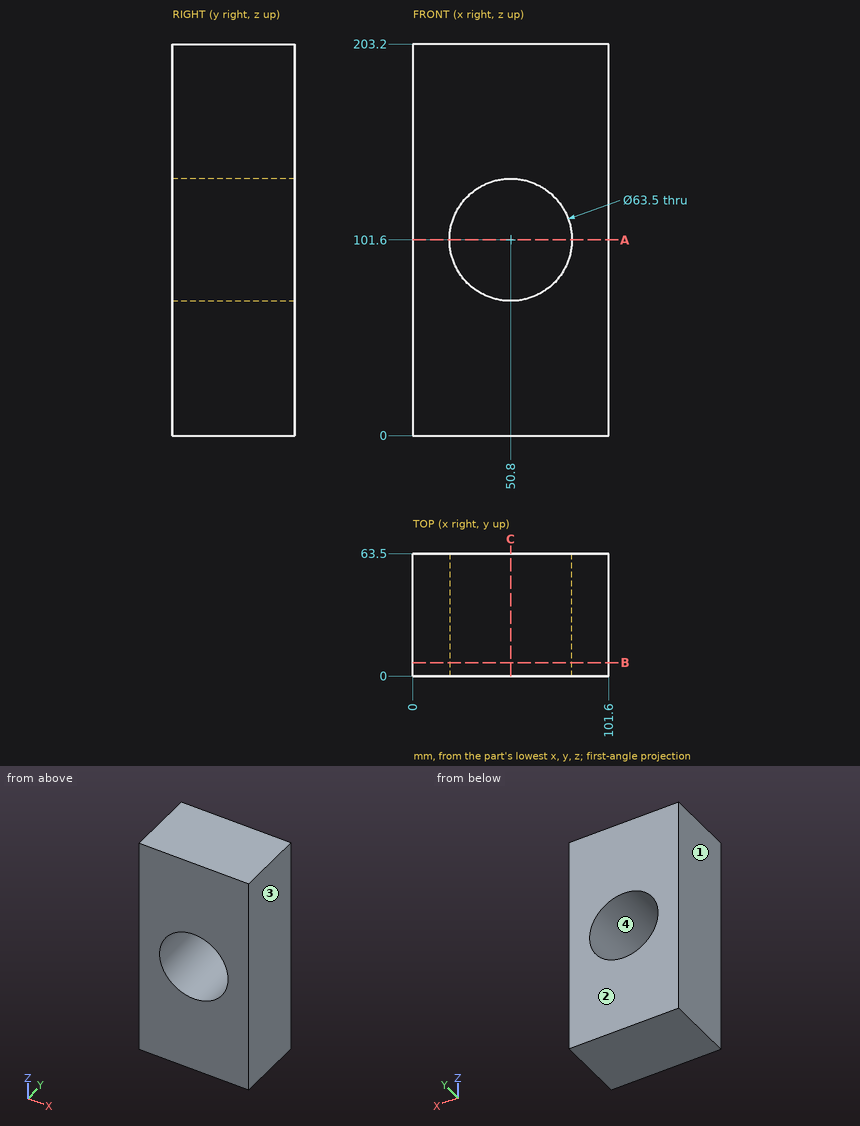
Design review of the part shown in the three views and the two pictorial views. Dimensions are in mm from the part's minimum x, y and z. Give positions to 0.01 mm unless a question says otherwise; leave off trailing zeros. Loops run counter-clockwise (first coordinate to the right, second up) from the corner with the lowest first, then second, coordinate; pieces in that order, holes last. Notation, with made-up numbers: M 31.25,48 L 73.25,48 A18 ccw 73.25,66 Z; hole C 89.25,68 d11. An arc over 180 degrees is marked long. Put each result on its own line as item: value. Start each with the question number.
(1) Wall thickness on L1, parallel to Z at x = 50.8, y = 39; L2, parallel to X at y = 48.5, z = 101.6; L3, parallel to Z at x = 32, y = 10: over which ranges is each line inside the solid? List them lowest first.
(2) Add section B-B, the plane y = 7. Write out the cut boundary in (x, z), then the cut area to 3 significant figures.
(3) For pin 1 (6 mm diameter, centred on x = 27.5, z = 164, fed in from -Y), flat-tipped, find the tip position at first contact; note if it passes through.
(4) Add section C-C, the plane x = 50.8. Write out the cut boundary in (y, z), then the cut area to 3 significant figures.
(5) The part is to be moulded in two halves that separate along X. For the marked faces 1, 2, 3 and 4, say which applies: +X half, -X half, draft (parallel to the pull), parting line (faces both ways), or undercut.
(6) Add section A-A, the plane z = 101.6. Write out the cut boundary in (x, y), then the cut area to 3 significant figures.
Result:
1. L1: z = 0 to 69.85, 133.35 to 203.2
1. L2: x = 0 to 19.05, 82.55 to 101.6
1. L3: z = 0 to 76.01, 127.19 to 203.2
2. outline: M 0,0 L 101.6,0 L 101.6,203.2 L 0,203.2 Z; hole C 50.8,101.6 d63.5
2. area: 17,500 mm^2
3. pin 1: stops at y = 0
4. outline: M 0,0 L 63.5,0 L 63.5,69.85 L 0,69.85 Z; M 0,133.35 L 63.5,133.35 L 63.5,203.2 L 0,203.2 Z
4. area: 8,870 mm^2
5. face 1: -X half
5. face 2: draft
5. face 3: +X half
5. face 4: undercut
6. outline: M 0,0 L 19.05,0 L 19.05,63.5 L 0,63.5 Z; M 82.55,0 L 101.6,0 L 101.6,63.5 L 82.55,63.5 Z
6. area: 2,420 mm^2
